Verification items for the finished model (mm, model axes). Face numbers are marked on the shaded views. A direction names the side the tool comes from. Give positions to 0.01 mm unless a question says otherwise; leave off trailing zeros. Loops run counter-clockwise (first coordinate to the right, second up) from the corner with the lowest first, then second, coordinate; pieces in that order, holes last. Notation, with made-up numbers: (-29, 17.25) - (-1, 17.25) arc R26 cw to (-1, 34.25) - close; hole circle Ø2 at (-2.5, -15.75). An arc over 180 degrees is marked (long way). Answer in a Markdown table with one row per item.
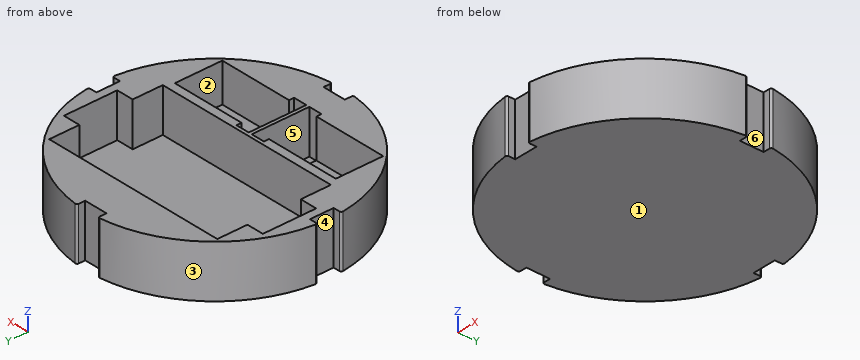
```python
from build123d import *

# Parameters (mm, degrees)
SKETCH2_R           = 75.692
BOSS_EXTRUDE1_DEPTH = 25.908
SKETCH3_R           = 75.692
BOSS_EXTRUDE2_DEPTH = 5.08
SKETCH4_W           = 44
SKETCH4_H           = 28
BOSS_EXTRUDE3_DEPTH = 3.048
CUT_EXTRUDE1_DEPTH  = 31.988
FILLET1_R           = 1.016


with BuildPart() as part:
    # Sketch2 → Boss-Extrude1 (new body)
    with BuildSketch(Plane.XY):
        Circle(SKETCH2_R)
        Polygon((-55.372, 48.26), (55.372, 48.26), (55.372, 30.48), (65.532, 30.48), (65.532, -1.016), (55.372, -1.016), (55.372, -18.796), (-55.372, -18.796), (-55.372, -1.016), (-65.532, -1.016), (-65.532, 30.48), (-55.372, 30.48), align=None, mode=Mode.SUBTRACT)
        Polygon((-53, -23.796), (-9, -23.796), (-9, -20.796), (-1, -20.796), (-1, -54.796), (-9, -54.796), (-9, -51.796), (-53, -51.796), align=None, mode=Mode.SUBTRACT)
        Polygon((53, -23.796), (9, -23.796), (9, -20.796), (1, -20.796), (1, -54.796), (9, -54.796), (9, -51.796), (53, -51.796), align=None, mode=Mode.SUBTRACT)
    extrude(amount=BOSS_EXTRUDE1_DEPTH)

    # Sketch3 → Boss-Extrude2 (add)
    with BuildSketch(Plane(origin=(0, 0, 0), x_dir=(-1, 0, 0), z_dir=(0, 0, -1))):
        Circle(SKETCH3_R)
    extrude(amount=BOSS_EXTRUDE2_DEPTH)

    # Sketch4 → Boss-Extrude3 (add)
    with BuildSketch(Plane.XY):
        with Locations((-31, -37.796)):
            Rectangle(SKETCH4_W, SKETCH4_H)
        with Locations((31, -37.796)):
            Rectangle(SKETCH4_W, SKETCH4_H)
    extrude(amount=BOSS_EXTRUDE3_DEPTH)

    # Sketch7 → Cut-Extrude1 (cut, through all)
    with BuildSketch(Plane.XY.offset(25.908)):
        with BuildLine():
            Line((6.985, 70.358), (-6.985, 70.358))
            Line((-6.985, 70.358), (-6.985, 75.369016439))
            ThreePointArc((-6.985, 75.369016439), (0, 75.692), (6.985, 75.369016439))
            Line((6.985, 75.369016439), (6.985, 70.358))
        make_face()
        with BuildLine():
            Line((70.358, -6.985), (70.358, 6.985))
            Line((70.358, 6.985), (75.369016439, 6.985))
            ThreePointArc((75.369016439, 6.985), (75.692, 0), (75.369016439, -6.985))
            Line((75.369016439, -6.985), (70.358, -6.985))
        make_face()
        with BuildLine():
            Line((-6.985, -70.358), (6.985, -70.358))
            Line((6.985, -70.358), (6.985, -75.369016439))
            ThreePointArc((6.985, -75.369016439), (0, -75.692), (-6.985, -75.369016439))
            Line((-6.985, -75.369016439), (-6.985, -70.358))
        make_face()
        with BuildLine():
            Line((-70.358, 6.985), (-70.358, -6.985))
            Line((-70.358, -6.985), (-75.369016439, -6.985))
            ThreePointArc((-75.369016439, -6.985), (-75.692, 0), (-75.369016439, 6.985))
            Line((-75.369016439, 6.985), (-70.358, 6.985))
        make_face()
    extrude(amount=-CUT_EXTRUDE1_DEPTH, mode=Mode.SUBTRACT)

    # Fillet1
    fillet1_edges = [part.edges().sort_by_distance(p)[0] for p in [
        (6.985, 75.369016439, 10.414),
        (-6.985, 75.369016439, 10.414),
        (75.369016439, -6.985, 10.414),
        (75.369016439, 6.985, 10.414),
        (-6.985, -75.369016439, 10.414),
        (6.985, -75.369016439, 10.414),
        (-75.369016439, 6.985, 10.414),
        (-75.369016439, -6.985, 10.414),
    ]]
    fillet(fillet1_edges, radius=FILLET1_R)


solid = part.part
```
Q1. Sectioned sample at A-A (x = 4). Record the cut outline in (y, z), and give its area (3 significant figures).
Completed:
| item | result |
|---|---|
| outline | (-70.36, -5.08) - (70.36, -5.08) - (70.36, 25.91) - (48.26, 25.91) - (48.26, 0) - (-18.8, 0) - (-18.8, 25.91) - (-20.8, 25.91) - (-20.8, 0) - (-54.8, 0) - (-54.8, 25.91) - (-70.36, 25.91) - close |
| area | 1,740 mm^2 |
Q2. Sectioned sample at C-C (y = 4). Record the cut outline in (x, z), and give its area (3 significant figures).
Completed:
| item | result |
|---|---|
| outline | (-70.36, -5.08) - (70.36, -5.08) - (70.36, 25.91) - (65.53, 25.91) - (65.53, 0) - (-65.53, 0) - (-65.53, 25.91) - (-70.36, 25.91) - close |
| area | 965 mm^2 |
Q3. Draft check along X on the marked faces 1, 2 and 3. Enter one of: +X half, -X half, draft (parallel to the pull), parting line (faces both ways), or undercut.
Completed:
| item | result |
|---|---|
| face 1 | draft |
| face 2 | undercut |
| face 3 | -X half |
Q4. Go/stop test with flat-tipped pins: P1, Ø2, axis at y = 48.5, z = -2, coming from the +X side; P2, Ø14, axis at y = -6, z = 18.5, coming from the -X side; P3, Ø5, axis at x = 42, z = 3, coming from the +Y side; P4, Ø6.5, axis at x = 3.5, z = 7, coming from the +Y side. Record where each tip stops, or that it passes through.
Completed:
| item | result |
|---|---|
| P1 | x = 58.93 |
| P2 | x = -75.26 |
| P3 | y = 64.57 |
| P4 | y = 70.36 |
Q5. Tool access check on the marked faces 4, 5 and 6. Record the directions out of +Z, -Z, +X, -X, +Y, -Y that give a thin tool (end or side, any length) a straight path to the whole face; none if there is none.
Completed:
| item | result |
|---|---|
| face 4 | +Z, -Z, -X |
| face 5 | +Z |
| face 6 | +Z, -Z, +X |
Q6. Thickness scan on line 1 (Y direction, x = -28, z = 14.5); line 2 (Y direction, x = 6.5, z = 10); line 3 (X direction, y = -37, z = 10). Record the ranges inside material, lowest first.
Completed:
| item | result |
|---|---|
| line 1 | -70.32 to -51.8, -23.8 to -18.8, 48.26 to 70.32 |
| line 2 | -70.36 to -54.8, -20.8 to -18.8, 48.26 to 70.36 |
| line 3 | -66.03 to -53, -1 to 1, 53 to 66.03 |
Q7. Sectioned sample at B-B (z = -3). Record the cut outline in (x, y) (3 decimals), and give its area (3 significant figures).
Completed:
| item | result |
|---|---|
| outline | (-75.256, -8.11) arc R75.692 ccw to (-8.11, -75.256) arc R1.016 ccw to (-6.985, -74.246) - (-6.985, -70.358) - (6.985, -70.358) - (6.985, -74.246) arc R1.016 ccw to (8.11, -75.256) arc R75.692 ccw to (75.256, -8.11) arc R1.016 ccw to (74.246, -6.985) - (70.358, -6.985) - (70.358, 6.985) - (74.246, 6.985) arc R1.016 ccw to (75.256, 8.11) arc R75.692 ccw to (8.11, 75.256) arc R1.016 ccw to (6.985, 74.246) - (6.985, 70.358) - (-6.985, 70.358) - (-6.985, 74.246) arc R1.016 ccw to (-8.11, 75.256) arc R75.692 ccw to (-75.256, 8.11) arc R1.016 ccw to (-74.246, 6.985) - (-70.358, 6.985) - (-70.358, -6.985) - (-74.246, -6.985) arc R1.016 ccw to start |
| area | 17,700 mm^2 |
Q8. Sectioned sample at D-D (z = 18). Give the number of separate pieces and of enclosed holes in the cut face, and give its area (3 significant figures).
Completed:
| item | result |
|---|---|
| separate pieces | 1 |
| enclosed holes | 3 |
| area | 6,630 mm^2 |
